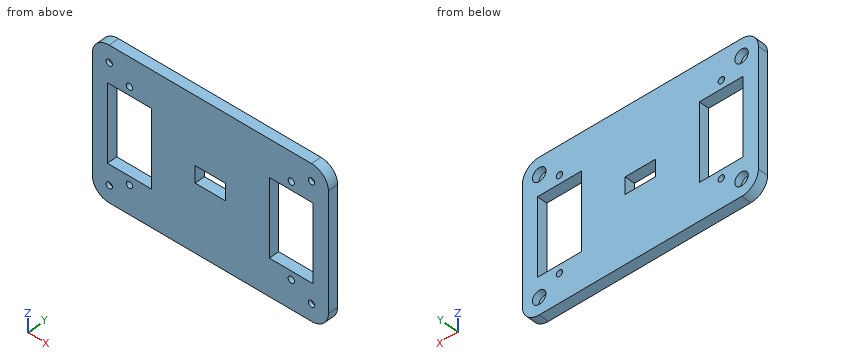
from build123d import *

# Parameters (mm, degrees)
SKETCH_1_W          = 70
SKETCH_1_H          = 45
EXTRUDE_1_DEPTH     = 3
SKETCH_2_W          = 13
SKETCH_2_H          = 23
CUT_EXTRUDE_1_DEPTH = 10
SKETCH_3_R          = 0.95
CUT_EXTRUDE_2_DEPTH = 10
FILLET_1_R          = 5
FILLET_2_R          = 5
SKETCH_4_R          = 0.95
CUT_EXTRUDE_3_DEPTH = 10
SKETCH_5_R          = 2
CUT_EXTRUDE_4_DEPTH = 2
SKETCH_6_W          = 9
SKETCH_6_H          = 5
CUT_EXTRUDE_5_DEPTH = 14


with BuildPart() as part:
    # 草图1 → 凸台-拉伸1 (new body)
    with BuildSketch(Plane(origin=(0, 0, 0), x_dir=(1, 0, 0), z_dir=(0, 1, 0))):
        Rectangle(SKETCH_1_W, SKETCH_1_H)
    extrude(amount=EXTRUDE_1_DEPTH)

    # 草图2 → 切除-拉伸1 (cut)
    with BuildSketch(Plane(origin=(0, 3, 0), x_dir=(1, 0, 0), z_dir=(0, 1, 0))):
        with Locations((24, 0)):
            Rectangle(SKETCH_2_W, SKETCH_2_H)
        with Locations((-24, 0)):
            Rectangle(SKETCH_2_W, SKETCH_2_H)
    extrude(amount=-CUT_EXTRUDE_1_DEPTH, mode=Mode.SUBTRACT)

    # 草图3 → 切除-拉伸2 (cut)
    with BuildSketch(Plane(origin=(0, 3, 0), x_dir=(1, 0, 0), z_dir=(0, 1, 0))):
        with Locations((-24, 14)):
            Circle(SKETCH_3_R)
        with Locations((-24, -14)):
            Circle(SKETCH_3_R)
        with Locations((24, 14)):
            Circle(SKETCH_3_R)
        with Locations((24, -14)):
            Circle(SKETCH_3_R)
    extrude(amount=-CUT_EXTRUDE_2_DEPTH, mode=Mode.SUBTRACT)

    # 圆角1
    fillet_1_edges = [part.edges().sort_by_distance(p)[0] for p in [
        (35, 1.5, -22.5),
    ]]
    fillet(fillet_1_edges, radius=FILLET_1_R)

    # 圆角2
    fillet_2_edges = [part.edges().sort_by_distance(p)[0] for p in [
        (35, 1.5, 22.5),
        (-35, 1.5, 22.5),
        (-35, 1.5, -22.5),
    ]]
    fillet(fillet_2_edges, radius=FILLET_2_R)

    # 草图4 → 切除-拉伸3 (cut)
    with BuildSketch(Plane(origin=(0, 3, 0), x_dir=(1, 0, 0), z_dir=(0, 1, 0))):
        with Locations((-30, 17.5)):
            Circle(SKETCH_4_R)
        with Locations((30, 17.5)):
            Circle(SKETCH_4_R)
        with Locations((-30, -17.5)):
            Circle(SKETCH_4_R)
        with Locations((30, -17.5)):
            Circle(SKETCH_4_R)
    extrude(amount=-CUT_EXTRUDE_3_DEPTH, mode=Mode.SUBTRACT)

    # 草图5 → 切除-拉伸4 (cut)
    with BuildSketch(Plane(origin=(0, 3, 0), x_dir=(1, 0, 0), z_dir=(0, 1, 0))):
        with Locations((-30, 17.5)):
            Circle(SKETCH_5_R)
        with Locations((30, 17.5)):
            Circle(SKETCH_5_R)
        with Locations((-30, -17.5)):
            Circle(SKETCH_5_R)
        with Locations((30, -17.5)):
            Circle(SKETCH_5_R)
    extrude(amount=-CUT_EXTRUDE_4_DEPTH, mode=Mode.SUBTRACT)

    # 草图6 → 切除-拉伸5 (cut)
    with BuildSketch(Plane(origin=(0, 3, 0), x_dir=(1, 0, 0), z_dir=(0, 1, 0))):
        Rectangle(SKETCH_6_W, SKETCH_6_H)
    extrude(amount=-CUT_EXTRUDE_5_DEPTH, mode=Mode.SUBTRACT)


solid = part.part
Design review of the part built by this model. Coordinates are the model's own, in mm. Coordinates: 2 decimals unless noted, no trailing zeros. Order: outer loops, then holes, each group sorted by start corner. A loop starts at its lowest first (then second) coordinate and runs counter-clockwise, first axis right, second up.
Item 1: For pin 1 Ø6 at (x, z) = (13.5, 12) entering from -Y; pin 2 Ø2.5 at (x, z) = (-30, 17.5) entering from +Y, all flat-tipped, find the tip position at first contact; note any pin that passes through.
Item 2: Take a section at C-C, the plane y = 1.55. Count the separate pieces of the cut face and the enclosed holes in it, then the cut area to 3 significant figures.
Item 3: For line 1 (X direction, y = 0.55, z = 7); line 2 (Z direction, x = 30, y = 0.7); line 3 (X direction, y = 2, z = -17.5), list the stretches that pass through material, from the lowest coordinate up.
Item 4: Take a section at B-B, the plane z = -10. Write out the cut boundary in (x, y), then the cut area to 3 significant figures.
Item 5: Take a section at D-D, the plane x = 21. Write out the cut boundary in (y, z), then the cut area to 3 significant figures.
Item 6: Take a section at A-A, the plane z = -1. Write out the cut boundary in (x, y), then the cut area to 3 significant figures.
The answers:
1. pin 1: stops at y = 0
1. pin 2: stops at y = 1
2. separate pieces: 1
2. enclosed holes: 11
2. area: 2,420 mm2
3. line 1: x = -35 to -30.5, -17.5 to 17.5, 30.5 to 35
3. line 2: z = -22.5 to -18.45, -16.55 to -11.5, 11.5 to 16.55, 18.45 to 22.5
3. line 3: x = -35 to -32, -28 to 28, 32 to 35
4. outline: (-35, 0) - (-30.5, 0) - (-30.5, 3) - (-35, 3) - close; (-17.5, 0) - (17.5, 0) - (17.5, 3) - (-17.5, 3) - close; (30.5, 0) - (35, 0) - (35, 3) - (30.5, 3) - close
4. area: 132 mm2
5. outline: (0, -22.5) - (3, -22.5) - (3, -11.5) - (0, -11.5) - close; (0, 11.5) - (3, 11.5) - (3, 22.5) - (0, 22.5) - close
5. area: 66.0 mm2
6. outline: (-35, 0) - (-30.5, 0) - (-30.5, 3) - (-35, 3) - close; (-17.5, 0) - (-4.5, 0) - (-4.5, 3) - (-17.5, 3) - close; (4.5, 0) - (17.5, 0) - (17.5, 3) - (4.5, 3) - close; (30.5, 0) - (35, 0) - (35, 3) - (30.5, 3) - close
6. area: 105 mm2
